from build123d import *

# Parameters (mm, degrees)
SKETCH1_R          = 20
EXTRUDE1_DEPTH     = 10
SKETCH2_R          = 30
CUT_EXTRUDE1_DEPTH = 7


with BuildPart() as part:
    # Sketch1 → Extrude1 (new, symmetric)
    with BuildSketch(Plane.XY):
        with BuildLine():
            Line((0, 50), (-625, 50))
            ThreePointArc((-625, 50), (-675, 0), (-625, -50))
            Line((-625, -50), (0, -50))
            ThreePointArc((0, -50), (50, 0), (0, 50))
        make_face()
        Circle(SKETCH1_R, mode=Mode.SUBTRACT)
        with Locations((-625, 0)):
            Circle(SKETCH1_R, mode=Mode.SUBTRACT)
    extrude(amount=EXTRUDE1_DEPTH, both=True)

    # Sketch2 → Cut-Extrude1 (cut)
    with BuildSketch(Plane.XY.offset(10)):
        with BuildLine():
            Line((0, 45), (-625, 45))
            ThreePointArc((-625, 45), (-670, 0), (-625, -45))
            Line((-625, -45), (0, -45))
            ThreePointArc((0, -45), (45, 0), (0, 45))
        make_face()
        Circle(SKETCH2_R, mode=Mode.SUBTRACT)
        with Locations((-625, 0)):
            Circle(SKETCH2_R, mode=Mode.SUBTRACT)
    cut_extrude1 = extrude(amount=-CUT_EXTRUDE1_DEPTH, mode=Mode.SUBTRACT)

    # Mirror1: Cut-Extrude1 across plane
    add(cut_extrude1.mirror(Plane.XY), mode=Mode.SUBTRACT)


solid = part.part
Part model, mm, in its own coordinate system. A direction names the side the tool comes from. Give positions to 0.01 mm unless a question says otherwise; leave off trailing zeros. Loops run counter-clockwise (first coordinate to the right, second up) from the corner with the lowest first, then second, coordinate; pieces in that order, holes last. Notation, with made-up numbers: M 22.5,27.25 L 81.5,27.25 A29 ccw 81.5,55.25 Z; hole C 49.25,53 d5. An arc over 180 degrees is marked long. Put each result on its own line as item: value. Start each with the question number.
1) Saw through at A-A (z = 6.5). List the corners of the cut face in (x, y), then the cut area to 3 significant figures.
2) Saw through at B-B (x = -568.5). List the corners of the cut face in (y, z).
3) Pull direction Y, two halves, no side cores. Call faces 1 (the flat face through (20, -6, 10)), 2 (the cylindrical face through (-29.97, 1.32, 6.55)), 3 (the cylindrical face through (49.988, -1.099, 0.14)), 4 (the cylindrical face through (-644.98, 0.88, -0.14)): +Y half, -Y half, draft (parallel to the pull), parting line (faces both ways), or undercut.
4) 3-axis set-ups, long thin cutter, end or side, ignore diameter. For faces 5 (the cylindrical face through (-597.288, -11.49, 6.549)), 6 (the flat face through (-605, -6, 10)), 7 (the flat face through (-318, 1, -3)): which of +Z, -Z, +X, -X, +Y, -Y reach the whole face in a straight line?
5) Flat gauge pins, fed straight in: pin 1 (3 mm diameter, centred on x = -435, y = 32.5, fed in from -Z); pin 2 (1 mm diameter, centred on y = -6, z = -5, fed in from -X); pin 3 (5 mm diameter, centred on y = 18.5, z = -0.5, fed in from +X). Where does each tip first touch, or does it go through?
6) Probe probe 1 along Y at (x, z) = (-92, -7.75); probe 2 along Y at (x, z) = (-625, -5.25); probe 3 along X at (y, z) = (-5, -3.75). List the from-to ranges inside material, lowest first.
7) Saw through at C-C (y = 0). State how many separate pieces and enclosed holes the cut face has, then the cut area to 3 significant figures.
Numbers:
1. outline: C -625,0 d60; M -625,-50 L 0,-50 A50 ccw 0,50 L -625,50 A50 ccw Z; C 0,0 d60; hole C -625,0 d40; hole M -625,-45 L 0,-45 A45 ccw 0,45 L -625,45 A45 ccw Z; hole C 0,0 d40
1. area: 10,900 mm^2
2. outline: M -50,-10 L -45,-10 L -45,-3 L 45,-3 L 45,-10 L 50,-10 L 50,10 L 45,10 L 45,3 L -45,3 L -45,10 L -50,10 Z
3. face 1: draft
3. face 2: undercut
3. face 3: parting line
3. face 4: undercut
4. face 5: +Z
4. face 6: +Z, +X, -X, +Y, -Y
4. face 7: -Z
5. pin 1: z = -3
5. pin 2: x = -674.7
5. pin 3: x = 47.37
6. probe 1: -50 to -45, 45 to 50
6. probe 2: -50 to -45, -30 to -20, 20 to 30, 45 to 50
6. probe 3: -674.75 to -669.72, -654.58 to -644.36, -605.64 to -595.42, -29.58 to -19.36, 19.36 to 29.58, 44.72 to 49.75
7. separate pieces: 3
7. enclosed holes: 0
7. area: 4,570 mm^2
